The listing builds one solid part. Answer for the finished solid, in the listing's coordinates (mm). A direction names the side the tool comes from. Give positions to 0.01 mm unless a question says otherwise; leave off trailing zeros. Loops run counter-clockwise (first coordinate to the right, second up) from the corner with the lowest first, then second, coordinate; pieces in that order, holes last. Notation, with made-up numbers: M 34.5,-11 L 76.5,-11 A10 ccw 76.5,5 Z; hole C 74,-3 d10. An arc over 180 degrees is marked long. One line per item, written item: value. Start each with the question number.
Q1. A cutting plane is placed at D-D, the plane x = -20. Determine the outline of the cut face in (y, z), and give its area (3 significant figures).
Q2. The mould has two halves that part along X. Classify faces 5 (the cylindrical face through (0.31, -0.6, -30.93)), 6 (the flat face through (19, 7, -1)), 7 (the flat face through (-12, 7, -1)), 8 (the cylindrical face through (-23.43, -0.6, -0.41)): +X half, -X half, draft (parallel to the pull), parting line (faces both ways), or undercut.
Q3. A cutting plane is placed at A-A, the plane x = -2.5. Determine the outline of the cut face in (y, z), and give its area (3 significant figures).
Q4. For faces 1 (the flat face through (0, -2, 9.5)), 2 (the cylindrical face through (-14.546, 11.05, -0.937)), 3 (the flat face through (12, 7, -1)), 4 (the flat face through (0, 0, 0)), determine the directions among +Z, -Z, +X, -X, +Y, -Y from which every point of the face is accessible in a straight line to the end or side of a thin tool.
Q5. A cutting plane is placed at B-B, the plane z = -22.5. Determine the outline of the cut face in (x, y).
Q6. A cutting plane is placed at C-C, the plane y = 2.75. Determine the outline of the cut face in (x, z), and give its area (3 significant figures).
Q7. Consider L1, parallel to Y at x = 15.5, z = 0.5; L2, parallel to Z at x = 14.5, y = 8.25; L3, parallel to Y at x = 15, z = -1. Determine where each line is inside the solid, lowest interval first.
Q8. Flat-ended cylindrical pins translate along their axes: pin 1 (4 mm diameter, centred on x = 16, y = 3, fed in from -Z); pin 2 (2.5 mm diameter, centred on y = 3.5, z = 1, fed in from -X); pin 3 (3 mm diameter, centred on x = -7.5, z = 2.5, fed in from +Y). Find the tip coordinate at first contact, or state that the pin passes through.
from build123d import *

# Parameters (mm, degrees)
CROQUIS1_W              = 48
CROQUIS1_H              = 63
CROQUIS1_R              = 5
SALIENTE_EXTRUIR1_DEPTH = 5
CROQUIS2_W              = 7
CROQUIS2_H              = 9
CROQUIS2_W_2            = 38
CROQUIS2_H_2            = 4
SALIENTE_EXTRUIR2_DEPTH = 13.5
CORTAR_EXTRUIR1_REACH   = 53.906
CROQUIS3_R              = 1.5
CORTAR_EXTRUIR2_REACH   = 46.534
CROQUIS4_R              = 1
REDONDEO1_R             = 2


with BuildPart() as part:
    # Croquis1 → Saliente-Extruir1 (new body)
    with BuildSketch(Plane(origin=(0, 0, 0), x_dir=(1, 0, 0), z_dir=(0, 1, 0))):
        Rectangle(CROQUIS1_W, CROQUIS1_H)
        with Locations(Location((-10.5, 22.5, 0), (0, 0, 270))):
            Circle(CROQUIS1_R, mode=Mode.SUBTRACT)
        with Locations(Location((10.5, 22.5, 0), (0, 0, 270))):
            Circle(CROQUIS1_R, mode=Mode.SUBTRACT)
        with BuildLine():
            Line((-9, -9.5), (9, -9.5))
            ThreePointArc((9, -9.5), (17, -17.5), (9, -25.5))
            Line((9, -25.5), (-9, -25.5))
            ThreePointArc((-9, -25.5), (-17, -17.5), (-9, -9.5))
        make_face(mode=Mode.SUBTRACT)
    extrude(amount=-SALIENTE_EXTRUIR1_DEPTH)

    # Croquis2 → Saliente-Extruir2 (add)
    with BuildSketch(Plane(origin=(0, 0, 0), x_dir=(1, 0, 0), z_dir=(0, 1, 0))):
        with Locations((15.5, 1)):
            Rectangle(CROQUIS2_W, CROQUIS2_H)
        with Locations((-15.5, 1)):
            Rectangle(CROQUIS2_W, CROQUIS2_H)
        with Locations((0, 14.5)):
            Rectangle(CROQUIS2_W_2, CROQUIS2_H_2)
    extrude(amount=SALIENTE_EXTRUIR2_DEPTH)

    # Croquis3 → Cortar-Extruir1 (cut, up to next)
    with BuildSketch(Plane.XY.offset(-12.5), mode=Mode.PRIVATE) as cortar_extruir1_sk1:
        with Locations((4.75, 6.75)):
            Circle(CROQUIS3_R)
    cortar_extruir1_tool1 = extrude(cortar_extruir1_sk1.sketch, amount=-CORTAR_EXTRUIR1_REACH, mode=Mode.PRIVATE) & part.part
    # Croquis3 → Cortar-Extruir1 (cut, up to next)
    with BuildSketch(Plane.XY.offset(-12.5), mode=Mode.PRIVATE) as cortar_extruir1_sk2:
        with Locations((-4.75, 6.75)):
            Circle(CROQUIS3_R)
    cortar_extruir1_tool2 = extrude(cortar_extruir1_sk2.sketch, amount=-CORTAR_EXTRUIR1_REACH, mode=Mode.PRIVATE) & part.part
    add(cortar_extruir1_tool1.solids().sort_by_distance((4.75, 6.75, -12.5))[0], mode=Mode.SUBTRACT)
    add(cortar_extruir1_tool2.solids().sort_by_distance((-4.75, 6.75, -12.5))[0], mode=Mode.SUBTRACT)

    # Croquis4 → Cortar-Extruir2 (cut, up to next)
    with BuildSketch(Plane.XY.offset(3.5), mode=Mode.PRIVATE) as cortar_extruir2_sk1:
        with Locations((15.5, 6.75)):
            Circle(CROQUIS4_R)
    cortar_extruir2_tool1 = extrude(cortar_extruir2_sk1.sketch, amount=-CORTAR_EXTRUIR2_REACH, mode=Mode.PRIVATE) & part.part
    # Croquis4 → Cortar-Extruir2 (cut, up to next)
    with BuildSketch(Plane.XY.offset(3.5), mode=Mode.PRIVATE) as cortar_extruir2_sk2:
        with Locations((15.5, 2.75)):
            Circle(CROQUIS4_R)
    cortar_extruir2_tool2 = extrude(cortar_extruir2_sk2.sketch, amount=-CORTAR_EXTRUIR2_REACH, mode=Mode.PRIVATE) & part.part
    # Croquis4 → Cortar-Extruir2 (cut, up to next)
    with BuildSketch(Plane.XY.offset(3.5), mode=Mode.PRIVATE) as cortar_extruir2_sk3:
        with Locations((15.5, 10.75)):
            Circle(CROQUIS4_R)
    cortar_extruir2_tool3 = extrude(cortar_extruir2_sk3.sketch, amount=-CORTAR_EXTRUIR2_REACH, mode=Mode.PRIVATE) & part.part
    # Croquis4 → Cortar-Extruir2 (cut, up to next)
    with BuildSketch(Plane.XY.offset(3.5), mode=Mode.PRIVATE) as cortar_extruir2_sk4:
        with Locations((-15.5, 2.75)):
            Circle(CROQUIS4_R)
    cortar_extruir2_tool4 = extrude(cortar_extruir2_sk4.sketch, amount=-CORTAR_EXTRUIR2_REACH, mode=Mode.PRIVATE) & part.part
    # Croquis4 → Cortar-Extruir2 (cut, up to next)
    with BuildSketch(Plane.XY.offset(3.5), mode=Mode.PRIVATE) as cortar_extruir2_sk5:
        with Locations((-15.5, 6.75)):
            Circle(CROQUIS4_R)
    cortar_extruir2_tool5 = extrude(cortar_extruir2_sk5.sketch, amount=-CORTAR_EXTRUIR2_REACH, mode=Mode.PRIVATE) & part.part
    # Croquis4 → Cortar-Extruir2 (cut, up to next)
    with BuildSketch(Plane.XY.offset(3.5), mode=Mode.PRIVATE) as cortar_extruir2_sk6:
        with Locations((-15.5, 10.75)):
            Circle(CROQUIS4_R)
    cortar_extruir2_tool6 = extrude(cortar_extruir2_sk6.sketch, amount=-CORTAR_EXTRUIR2_REACH, mode=Mode.PRIVATE) & part.part
    add(cortar_extruir2_tool1.solids().sort_by_distance((15.5, 6.75, 3.5))[0], mode=Mode.SUBTRACT)
    add(cortar_extruir2_tool2.solids().sort_by_distance((15.5, 2.75, 3.5))[0], mode=Mode.SUBTRACT)
    add(cortar_extruir2_tool3.solids().sort_by_distance((15.5, 10.75, 3.5))[0], mode=Mode.SUBTRACT)
    add(cortar_extruir2_tool4.solids().sort_by_distance((-15.5, 2.75, 3.5))[0], mode=Mode.SUBTRACT)
    add(cortar_extruir2_tool5.solids().sort_by_distance((-15.5, 6.75, 3.5))[0], mode=Mode.SUBTRACT)
    add(cortar_extruir2_tool6.solids().sort_by_distance((-15.5, 10.75, 3.5))[0], mode=Mode.SUBTRACT)

    # Redondeo1
    redondeo1_edges = [part.edges().sort_by_distance(p)[0] for p in [
        (-24, -5, 0),
        (0, -5, 31.5),
        (24, -5, 0),
        (0, 0, 31.5),
        (-24, 0, 0),
        (0, 0, -31.5),
        (24, 0, 0),
        (24, -2.5, 31.5),
        (-24, -2.5, 31.5),
        (-24, -2.5, -31.5),
        (24, -2.5, -31.5),
        (0, -5, -31.5),
    ]]
    fillet(redondeo1_edges, radius=REDONDEO1_R)


solid = part.part
Answer block:
1. outline: M -5,-29.5 A2 ccw -3,-31.5 L -2,-31.5 A2 ccw 0,-29.5 L 0,29.5 A2 ccw -2,31.5 L -3,31.5 A2 ccw -5,29.5 Z
1. area: 312 mm^2
2. face 5: draft
2. face 6: +X half
2. face 7: undercut
2. face 8: -X half
3. outline: M -5,-29.5 A2 ccw -3,-31.5 L -2,-31.5 A2 ccw 0,-29.5 L 0,-16.5 L 13.5,-16.5 L 13.5,-12.5 L 0,-12.5 L 0,9.5 L -5,9.5 Z; M -5,25.5 L 0,25.5 L 0,29.5 A2 ccw -2,31.5 L -3,31.5 A2 ccw -5,29.5 Z
3. area: 286 mm^2
4. face 1: +Y, -Y
4. face 2: +Z
4. face 3: +Z, +Y
4. face 4: +Y
5. outline: M -24,-3 A2 ccw -22,-5 L -15.5,-5 L -15.5,0 L -22,0 A2 ccw -24,-2 Z; M -5.5,-5 L 5.5,-5 L 5.5,0 L -5.5,0 Z; M 15.5,-5 L 22,-5 A2 ccw 24,-3 L 24,-2 A2 ccw 22,0 L 15.5,0 Z
6. outline: M -19,-16.5 L 19,-16.5 L 19,-12.5 L -19,-12.5 Z; M -19,-5.5 L -16.5,-5.5 L -16.5,3.5 L -19,3.5 Z; M -14.5,-5.5 L -12,-5.5 L -12,3.5 L -14.5,3.5 Z; M 12,-5.5 L 14.5,-5.5 L 14.5,3.5 L 12,3.5 Z; M 16.5,-5.5 L 19,-5.5 L 19,3.5 L 16.5,3.5 Z
6. area: 242 mm^2
7. L1: -5 to 1.75, 3.75 to 5.75, 7.75 to 9.75, 11.75 to 13.5
7. L2: -16.5 to -12.5, -5.5 to 3.5
7. L3: -5 to 1.88, 3.62 to 5.88, 7.62 to 9.88, 11.62 to 13.5
8. pin 1: z = -16.5
8. pin 2: x = -19
8. pin 3: y = 0
